The model under review builds one solid part; all positions refer to its coordinate system, in mm. A direction names the side the tool comes from. Coordinates: 2 decimals unless noted, no trailing zeros. Order: outer loops, then holes, each group sorted by start corner. A loop starts at its lowest first (then second) coordinate and runs counter-clockwise, first axis right, second up.
```python
from build123d import *

# Parameters (mm, degrees)
F0_W     = 77.5483176112
F0_H     = 138.3502483368
F1_DEPTH = 25.4
F2_W     = 25.4
F2_H     = 25.4218988121
F3_DEPTH = 48.006
F4_R     = 5.08
F5_DEPTH = 50.8
F6_DEPTH = 50.8
F7_DEPTH = 50.8


with BuildPart() as f1:
    # F0 (on Front) → F1 (new body)
    with BuildSketch(Plane.XZ):
        with Locations((-29.2568616569, 0.0140890479)):
            Rectangle(F0_W, F0_H)
    extrude(amount=F1_DEPTH)

    # F2 (on face) → F3 (cut)
    with BuildSketch(Plane.YZ.offset(9.5172971487)):
        with Locations((-12.7, 33.0090541393)):
            Rectangle(F2_W, F2_H)
        with Locations((-12.7, -27.8852600604)):
            Rectangle(F2_W, F2_H)
    extrude(amount=-F3_DEPTH, mode=Mode.SUBTRACT)

    # F4
    f4_edges = [f1.edges().sort_by_distance(p)[0] for p in [
        (9.517297, -25.4, 57.454608),
        (-14.485703, -25.4, 45.720004),
        (-38.488703, -25.4, 33.009054),
        (-14.485703, -25.4, 20.298105),
        (9.517297, -25.4, 2.561897),
        (-14.485703, -25.4, -15.174311),
        (-38.488703, -25.4, -27.88526),
        (-14.485703, -25.4, -40.596209),
        (9.517297, -25.4, -54.878622),
        (-29.256862, -25.4, -69.161035),
        (-68.03102, -25.4, 0.014089),
        (-29.256862, -25.4, 69.189213),
        (9.517297, 0, 57.454608),
        (-14.485703, 0, 45.720004),
        (-38.488703, 0, 33.009054),
        (-14.485703, 0, 20.298105),
        (9.517297, 0, 2.561897),
        (-14.485703, 0, -15.174311),
        (-38.488703, 0, -27.88526),
        (-14.485703, 0, -40.596209),
        (9.517297, 0, -54.878622),
        (-29.256862, 0, -69.161035),
        (-68.03102, 0, 0.014089),
        (-29.256862, 0, 69.189213),
        (-68.03102, -12.7, 69.189213),
        (-68.03102, -12.7, -69.161035),
        (9.517297, -12.7, 69.189213),
        (9.517297, -12.7, 45.720004),
        (-38.488703, -12.7, 45.720004),
        (9.517297, -12.7, -15.174311),
        (-38.488703, -12.7, -15.174311),
        (9.517297, -12.7, 20.298105),
        (-38.488703, -12.7, 20.298105),
        (9.517297, -12.7, -69.161035),
        (9.517297, -12.7, -40.596209),
        (-38.488703, -12.7, -40.596209),
    ]]
    fillet(f4_edges, radius=F4_R)

    # F5 (cut): a face of the model
    f5_faces = [f1.faces().sort_by_distance(p)[0] for p in [
        (9.5172971487, -12.7, 57.4546083808),
    ]]
    extrude(f5_faces, amount=-F5_DEPTH, mode=Mode.SUBTRACT)

    # F6 (cut): a face of the model
    f6_faces = [f1.faces().sort_by_distance(p)[0] for p in [
        (9.5172971487, -12.7, 2.5618970394),
    ]]
    extrude(f6_faces, amount=-F6_DEPTH, mode=Mode.SUBTRACT)

    # F7 (cut): a face of the model
    f7_faces = [f1.faces().sort_by_distance(p)[0] for p in [
        (9.5172971487, -12.7, -54.8786222935),
    ]]
    extrude(f7_faces, amount=-F7_DEPTH, mode=Mode.SUBTRACT)


solid = f1.part
```
(1) We need section A-A, the plane x = -7. Count the separate pieces of the cut face and the enclosed holes in it, and give its area (3 significant figures).
A:
separate pieces: 3
enclosed holes: 3
area: 1,290 mm2
(2) Machinability: for faces 5 (the face through (-40.016, -23.951, -27.778)), 6 (the face through (-41.283, -13, 57)), 7 (the face through (-37.04, -12.59, -39.07)), which of the approach directions +Z, -Z, +X, -X, +Y, -Y give a long, thin tool a straight path to every point of the face, cutting with its end or side? Answer none if there is none.
A:
face 5: +X, -Y
face 6: +X
face 7: +X, +Y, -Y
(3) We need section B-B, the plane z = 34.5. Write out the cut boundary in (x, y), and give its area (3 significant figures).
A:
outline: (-68.03, -20.32) arc R5.08 ccw to (-62.95, -25.4) - (-43.57, -25.4) arc R5.08 ccw to (-38.49, -20.32) - (-38.49, -5.08) arc R5.08 ccw to (-43.57, 0) - (-62.95, 0) arc R5.08 ccw to (-68.03, -5.08) - close
area: 728 mm2
(4) For pin 1 Ø2 at (y, z) = (-18, -18) entering from +X; pin 2 Ø5 at (y, z) = (-20.5, 10.5) entering from -X; pin 3 Ø1 at (y, z) = (-19, 55) entering from +X; pin 4 Ø4 at (y, z) = (-8.5, 38) entering from +X, all flat-tipped, find the tip position at first contact; note any pin that passes through.
A:
pin 1: stops at x = -37.31
pin 2: stops at x = -68.03
pin 3: stops at x = -41.28
pin 4: stops at x = -38.49
(5) Wall thickness on probe 1 along Z at (x, y) = (-6, -9.25); probe 2 along Z at (x, y) = (-15, -5); probe 3 along Z at (x, y) = (-39, -18.25): over which ranges is each line inside the solid? List them lowest first.
A:
probe 1: z = -69.16 to -64.08, -45.68 to -40.6, -15.17 to -10.09, 15.22 to 20.3, 45.72 to 50.8, 64.11 to 69.19
probe 2: z = -69.16 to -40.6, -15.17 to 20.3, 45.72 to 69.19
probe 3: z = -69.16 to -64.08, -45.68 to -10.09, 15.22 to 50.8, 64.11 to 69.19
(6) Draft analysis for pull direction Z (two halves, no side actions). For faces 1 (the face through (-28.785, -1.528, 67.741)), 2 (the face through (-14.751, -23.951, 47.248)), 3 (the face through (-36.96, -12.59, 44.27)), 4 (the face through (7.99, -23.95, 2.74)), state which applies: released by +Z, released by -Z, zero draft, split by the parting line, or undercut.
A:
face 1: released by +Z
face 2: undercut
face 3: undercut
face 4: zero draft
(7) We need section D-D, the plane z = -54.5. Write out the cut boundary in (x, y).
A:
outline: (-68.03, -20.32) arc R5.08 ccw to (-62.95, -25.4) - (4.44, -25.4) arc R5.08 ccw to (9.52, -20.32) - (-41.28, -20.32) - (-41.28, -5.08) - (9.52, -5.08) arc R5.08 ccw to (4.44, 0) - (-62.95, 0) arc R5.08 ccw to (-68.03, -5.08) - close
